```python
from build123d import *

# Parameters (mm, degrees)
BOSS_EXTRUDE1_DEPTH         = 19.05
SKETCH3_R                   = 24.5745
CUT_EXTRUDE1_DEPTH          = 175.004260005
SKETCH5_R                   = 51.3715
SKETCH5_R_2                 = 46.5455
CUT_EXTRUDE2_DEPTH          = 2.794
SKETCH7_R                   = 4
CUT_EXTRUDE3_DEPTH          = 12.7
M8_TAPPED_HOLE1_D           = 6.8
M8_TAPPED_HOLE1_DEPTH       = 13.957067295
M8_TAPPED_HOLE1_CSINK_D     = 8.05
M8_TAPPED_HOLE1_CSINK_ANGLE = 90
M8_TAPPED_HOLE1_TIP         = 2.042926105
CIRPATTERN1_COUNT           = 8


with BuildPart() as part:
    # Sketch1 → Boss-Extrude1 (new body)
    with BuildSketch(Plane(origin=(0, 0, 0), x_dir=(1, 0, 0), z_dir=(0, 1, 0))):
        with BuildLine():
            ThreePointArc((-31.932272077, 122.3), (-48.371185851, 116.778372909), (-63.899633215, 109.058685463))
            Line((-63.899633215, 109.058685463), (-109.058685463, 63.899633215))
            ThreePointArc((-109.058685463, 63.899633215), (-116.778372909, 48.371185851), (-122.3, 31.932272077))
            Line((-122.3, 31.932272077), (-122.3, -31.932272077))
            ThreePointArc((-122.3, -31.932272077), (-116.778372909, -48.371185851), (-109.058685463, -63.899633215))
            Line((-109.058685463, -63.899633215), (-63.899633215, -109.058685463))
            ThreePointArc((-63.899633215, -109.058685463), (-48.371185851, -116.778372909), (-31.932272077, -122.3))
            Line((-31.932272077, -122.3), (31.932272077, -122.3))
            ThreePointArc((31.932272077, -122.3), (48.371185851, -116.778372909), (63.899633215, -109.058685463))
            Line((63.899633215, -109.058685463), (109.058685463, -63.899633215))
            ThreePointArc((109.058685463, -63.899633215), (116.778372909, -48.371185851), (122.3, -31.932272077))
            Line((122.3, -31.932272077), (122.3, 31.932272077))
            ThreePointArc((122.3, 31.932272077), (116.778372909, 48.371185851), (109.058685463, 63.899633215))
            Line((109.058685463, 63.899633215), (63.899633215, 109.058685463))
            ThreePointArc((63.899633215, 109.058685463), (48.371185851, 116.778372909), (31.932272077, 122.3))
            Line((31.932272077, 122.3), (-31.932272077, 122.3))
        make_face()
    extrude(amount=BOSS_EXTRUDE1_DEPTH)

    # Sketch3 → Cut-Extrude1 (cut, through all)
    with BuildSketch(Plane(origin=(0, 19.05, 0), x_dir=(1, 0, 0), z_dir=(0, 1, 0))):
        with Locations(Location((0, 0, 0), (0, 0, 270))):
            Circle(SKETCH3_R)
    extrude(amount=-CUT_EXTRUDE1_DEPTH, mode=Mode.SUBTRACT)

    # Sketch5 → Cut-Extrude2 (cut)
    with BuildSketch(Plane(origin=(0, 19.05, 0), x_dir=(1, 0, 0), z_dir=(0, 1, 0))):
        with Locations(Location((0, 0, 0), (0, 0, 270))):
            Circle(SKETCH5_R)
        with Locations(Location((0, 0, 0), (0, 0, 270))):
            Circle(SKETCH5_R_2, mode=Mode.SUBTRACT)
    extrude(amount=-CUT_EXTRUDE2_DEPTH, mode=Mode.SUBTRACT)

    # Sketch7 → Cut-Extrude3 (cut)
    with BuildSketch(Plane.XZ):
        with Locations(Location((-71.374, 0, 0), (0, 0, 270))):
            Circle(SKETCH7_R)
    cut_extrude3 = extrude(amount=-CUT_EXTRUDE3_DEPTH, mode=Mode.SUBTRACT)

    # M8 Tapped Hole1
    with Locations(Plane(origin=(0, 0, 0), x_dir=(-1, 0, 0), z_dir=(0, -1, 0))):
        with Locations((-71.374, 0)):
            CounterSinkHole(M8_TAPPED_HOLE1_D / 2, M8_TAPPED_HOLE1_CSINK_D / 2, depth=M8_TAPPED_HOLE1_DEPTH, counter_sink_angle=M8_TAPPED_HOLE1_CSINK_ANGLE)
            with Locations((0, 0, -(M8_TAPPED_HOLE1_DEPTH + M8_TAPPED_HOLE1_TIP / 2))):  # 118° drill point
                Cone(0, M8_TAPPED_HOLE1_D / 2, M8_TAPPED_HOLE1_TIP, mode=Mode.SUBTRACT)

    # CirPattern1: Cut-Extrude3 ×8 about axis
    cirpattern1_axis = Axis((0, 0, 0), (0, 1, 0))
    for i in range(1, CIRPATTERN1_COUNT):
        add(cut_extrude3.rotate(cirpattern1_axis, i * 360 / CIRPATTERN1_COUNT), mode=Mode.SUBTRACT)


solid = part.part
```
Could you check a few things on this model? Use its own coordinates, in mm. A direction names the side the tool comes from. Coordinates: 2 decimals unless noted, no trailing zeros. Loops run counter-clockwise (first coordinate to the right, second up) from the corner with the lowest first, then second, coordinate; pieces in that order, holes last. Notation, with made-up numbers: M -16,74 L 40,74 A24 cw 40,87 Z; hole C 0.25,24.25 d10. An arc over 180 degrees is marked long. Put each result on its own line as item: value. Start each with the question number.
(1) For faces 5 (the face through (0, 9, 122.3)), 6 (the face through (75, 12.7, -1)), 7 (the face through (38.3, 16.256, -26.9)), which set-ups out of +Z, -Z, +X, -X, +Y, -Y let a thin tool reach every point of the face, with its end or its side?
(2) Suppose I cut it at A-A on x = 0. Please give me the cut outline in (y, z), then the cut area to 3 significant figures.
(3) Suppose I cut it at D-D on z = 60. Please give me the cut outline in (x, y), then the cut area to 3 significant figures.
(4) Will these pins go through, and if not, where does the flat tip stop? P1, Ø8, axis at x = 87.5, y = 4.5, coming from the -Z side; P2, Ø5, axis at x = -50.47, z = -50.47, coming from the -Y side; P3, Ø5, axis at y = 10, z = 67, coming from the -X side.
(5) Suppose I cut it at B-B on z = 19. Please give me the cut outline in (x, y), then the cut area to 3 significant figures.
(6) Suppose I cut it at C-C on y = 5. Count the separate pieces of the cut face and the enclosed holes in it, then the cut area to 3 significant figures.
(7) Thinking about a two-plate mould opening in X: for faces 1 (the face through (-1.85, 6.26, 74.92)), 2 (the face through (86.16, 9.39, 86.8)), 3 (the face through (0, 9, -122.3)), 4 (the face through (-122.3, 9, 0)), which applies, pulls with the +X half, pulls with the -X half, needs draft (parallel to the pull), parting line crosses it, or undercut?
(8) I need wall thicknesses on line 1 (X direction, y = 12.25, z = -1); line 2 (Z direction, x = 33, y = 16.75); line 3 (Z direction, x = 8, y = 6). Which ranges of each line are inside material? Lowest first, please. Write a range as from..to.
Solutions:
1. face 5: +Z, +X, -X, +Y, -Y
1. face 6: -Y
1. face 7: +Y
2. outline: M 0,-122.3 L 19.05,-122.3 L 19.05,-51.37 L 16.26,-51.37 L 16.26,-46.55 L 19.05,-46.55 L 19.05,-24.57 L 0,-24.57 L 0,-67.37 L 12.7,-67.37 L 12.7,-75.37 L 0,-75.37 Z; M 0,24.57 L 19.05,24.57 L 19.05,46.55 L 16.26,46.55 L 16.26,51.37 L 19.05,51.37 L 19.05,122.3 L 0,122.3 L 0,75.37 L 12.7,75.37 L 12.7,67.37 L 0,67.37 Z
2. area: 3,490 mm2
3. outline: M -111.25,0 L 111.25,0 L 111.25,19.05 L -111.25,19.05 Z
3. area: 4,240 mm2
4. P1: stops at z = -89.46
4. P2: stops at y = 12.7
4. P3: stops at x = -108.46
5. outline: M -122.3,0 L -15.59,0 L -15.59,19.05 L -42.49,19.05 L -42.49,16.26 L -47.73,16.26 L -47.73,19.05 L -122.3,19.05 Z; M 15.59,0 L 122.3,0 L 122.3,19.05 L 47.73,19.05 L 47.73,16.26 L 42.49,16.26 L 42.49,19.05 L 15.59,19.05 Z
5. area: 4,040 mm2
6. separate pieces: 1
6. enclosed holes: 9
6. area: 46,500 mm2
7. face 1: undercut
7. face 2: pulls with the +X half
7. face 3: needs draft
7. face 4: pulls with the -X half
8. line 1: x = -122.3..-75.25, -67.5..-24.55, 24.55..67.5, 75.25..122.3
8. line 2: z = -122.02..-39.37, -32.83..32.83, 39.37..122.02
8. line 3: z = -122.3..-23.24, 23.24..122.3
